```python
from build123d import *

# Parameters (mm, degrees)
F1_DEPTH = 47.498


with BuildPart() as f1:
    # F0 (on Front) → F1 (new body)
    with BuildSketch(Plane.XZ):
        Polygon((-26.450716, 11.804912), (-13.750716, 11.804912), (-13.750716, 37.204912), (-39.150716, 37.204912), (-67.213629, 11.435105), (-89.950716, 37.204912), (-115.350716, 37.204912), (-115.350716, 11.804912), (-102.650716, 11.804912), (-102.650716, -13.595088), (-115.350716, -13.595088), (-115.350716, -64.395088), (-89.950716, -64.395088), (-89.950716, -38.995088), (-39.150716, -38.995088), (-39.150716, -64.395088), (-13.750716, -64.395088), (-13.750716, -13.595088), (-26.450716, -13.595088), align=None)
    extrude(amount=F1_DEPTH)


solid = f1.part
```
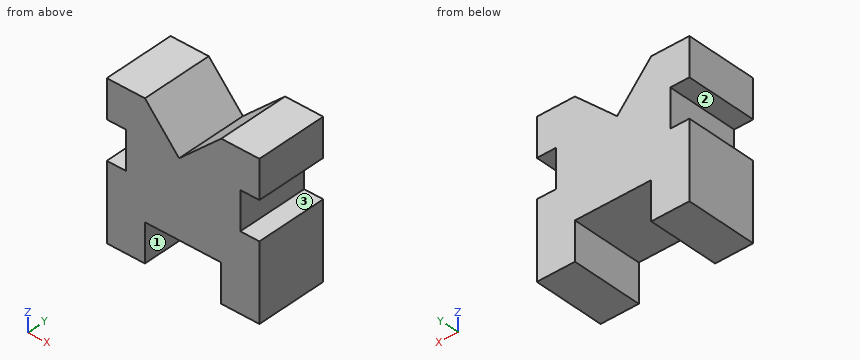
Design review of the part built by this model. Coordinates are the model's own, in mm. Face numbers are marked on the shaded views. A direction names the side the tool comes from. Coordinates: 2 decimals unless noted, no trailing zeros. Order: outer loops, then holes, each group sorted by start corner. A loop starts at its lowest first (then second) coordinate and runs counter-clockwise, first axis right, second up. Notation, with made-up numbers: M -25.5,78 L 11.5,78 A10 ccw 11.5,94 Z; hole C 29.5,-14.75 d1. An arc over 180 degrees is marked long. Answer as a JSON object with one key per item and string values. Group by question number.
1) Add section D-D, the plane z = -4. Write out the cut boundary in (x, y).
2) For pin 1 (1.5 mm diameter, centred on y = -40.5, z = 0, fed in from -X); pin 2 (20.5 mm diameter, centred on y = -29, z = 3, fed in from +X), all flat-tipped, find the tip position at first contact; note any pin that passes through.
3) Add section A-A, the plane z = -45. Write out the cut boundary in (x, y).
4) Add section C-C, the plane y = -33.5. Write out the cut boundary in (x, z).
5) Add section B-B, the plane x = -23.5. Write out the cut boundary in (y, z).
6) Tool access review of the marked faces 1, 2 and 3: name each direction out of +Z, -Z, +X, -X, +Y, -Y from which nothing blocks a thin tool from reaching the whole face with its end or side.
7) Wall thickness on L1, parallel to X at y = -6, z = -59; L2, parallel to Z at x = -103.5, y = -19.5; L3, parallel to X at y = -32, z = 14.5: over which ranges is each line inside the solid? List them lowest first.
Computed values:
{
 "1": {"outline": "M -102.65,-47.5 L -26.45,-47.5 L -26.45,0 L -102.65,0 Z"},
 "2": {"pin 1": "stops at x = -102.65", "pin 2": "stops at x = -13.75"},
 "3": {"outline": "M -115.35,-47.5 L -89.95,-47.5 L -89.95,0 L -115.35,0 Z; M -39.15,-47.5 L -13.75,-47.5 L -13.75,0 L -39.15,0 Z"},
 "4": {"outline": "M -115.35,-64.4 L -89.95,-64.4 L -89.95,-39 L -39.15,-39 L -39.15,-64.4 L -13.75,-64.4 L -13.75,-13.6 L -26.45,-13.6 L -26.45,11.8 L -13.75,11.8 L -13.75,37.2 L -39.15,37.2 L -67.21,11.44 L -89.95,37.2 L -115.35,37.2 L -115.35,11.8 L -102.65,11.8 L -102.65,-13.6 L -115.35,-13.6 Z"},
 "5": {"outline": "M -47.5,-64.4 L 0,-64.4 L 0,-13.6 L -47.5,-13.6 Z; M -47.5,11.8 L 0,11.8 L 0,37.2 L -47.5,37.2 Z"},
 "6": {"face 1": "-Z, +Y, -Y", "face 2": "-X, +Y, -Y", "face 3": "+X, +Y, -Y"},
 "7": {"L1": "x = -115.35 to -89.95, -39.15 to -13.75", "L2": "z = -64.4 to -13.6, 11.8 to 37.2", "L3": "x = -115.35 to -69.92, -63.88 to -13.75"}
}
